Design review of the part built by this model. Coordinates are the model's own, in mm. Face numbers are marked on the shaded views. Round coordinates to 2 decimals unless told otherwise and drop trailing zeros. Order: outer loops, then holes, each group sorted by start corner. A loop starts at its lowest first (then second) coordinate and runs counter-clockwise, first axis right, second up.
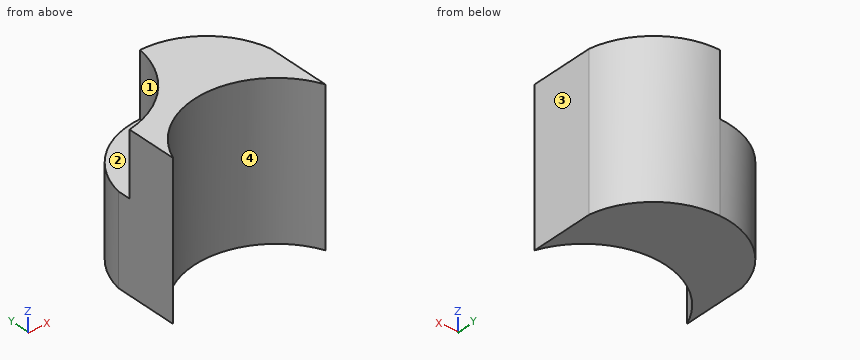
from build123d import *

# Parameters (mm, degrees)
SKETCH1_W           = 6
SKETCH1_H           = 6
BOSS_EXTRUDE1_DEPTH = 5
CUT_EXTRUDE4_DEPTH  = 12.5
CUT_EXTRUDE5_DEPTH  = 2.5


with BuildPart() as part:
    # Sketch1 → Boss-Extrude1 (new body)
    with BuildSketch(Plane(origin=(0, 0, 0), x_dir=(1, 0, 0), z_dir=(0, 1, 0))):
        Rectangle(SKETCH1_W, SKETCH1_H)
    extrude(amount=BOSS_EXTRUDE1_DEPTH)

    # Sketch5 → Cut-Extrude4 (cut)
    with BuildSketch(Plane.XY.offset(3)):
        with BuildLine():
            Line((-3, 5), (-3, 2.5))
            ThreePointArc((-3, 2.5), (-1.952562419, 4.293074903), (0, 5))
            Line((0, 5), (-3, 5))
        make_face()
        with BuildLine():
            ThreePointArc((0, 5), (1.952562419, 4.293074903), (3, 2.5))
            Line((3, 2.5), (3, 5))
            Line((3, 5), (0, 5))
        make_face()
        with BuildLine():
            ThreePointArc((-3, 0), (0, 2), (3, 0))
            Line((3, 0), (-3, 0))
        make_face()
    extrude(amount=-CUT_EXTRUDE4_DEPTH, mode=Mode.SUBTRACT)

    # Sketch6 → Cut-Extrude5 (cut)
    with BuildSketch(Plane.XY.offset(3)):
        with BuildLine():
            ThreePointArc((-3, 2), (-1.009831788, 3.009831788), (0, 5))
            ThreePointArc((0, 5), (-1.952562419, 4.293074903), (-3, 2.5))
            Line((-3, 2.5), (-3, 2))
        make_face()
    extrude(amount=-CUT_EXTRUDE5_DEPTH, mode=Mode.SUBTRACT)


solid = part.part
1) The part is to be moulded in two halves that separate along X. For the marked faces 1, 2, 3 and 4, say which applies: released by +X, released by -X, zero draft, split by the parting line, or undercut.
Results:
face 1: released by -X
face 2: zero draft
face 3: released by +X
face 4: undercut
2) To check wall thickness, follow line 1 along X through (y, z) = (1.1, 0.15) (3 decimals); line 2 along X through (y, z) = (1.55, 2.55); line 3 along Y through (x, z) = (2.5, -1.25). State the ranges of each line that lie inside material, in increasing order.
Results:
line 1: x = -3 to -2.245, 2.245 to 3
line 2: x = -3 to -1.65, 1.65 to 3
line 3: y = 0.83 to 3.7
3) Take a section at A-A on y = 0.4. Give the boundary of the cut face in (x, z).
Results:
outline: (-3, -3) - (-2.8, -3) - (-2.8, 3) - (-3, 3) - close; (2.8, -3) - (3, -3) - (3, 3) - (2.8, 3) - close
4) Take a section at B-B on z = -1. Give the boundary of the cut face in (x, y), plus the area to 3 significant figures.
Results:
outline: (-3, 0) arc R3.25 cw to (3, 0) - (3, 2.5) arc R3.05 ccw to (-3, 2.5) - close
area: 17.6 mm2
5) Take a section at D-D on y = 1.4. Give the boundary of the cut face in (x, z), plus the area to 3 significant figures.
Results:
outline: (-3, -3) - (-1.88, -3) - (-1.88, 3) - (-3, 3) - close; (1.88, -3) - (3, -3) - (3, 3) - (1.88, 3) - close
area: 13.4 mm2
6) Clearance check with a flat-ended pin moving along its axis: P1, Ø3, axis at x = 0.5, z = 1.5, coming from the -Y side. State where the tip first meets the part, or that it passes through.
Results:
P1: stops at y = 1.31
7) Take a section at C-C on x = -1. Give the boundary of the cut face in (y, z).
Results:
outline: (1.84, -3) - (4.83, -3) - (4.83, 0.5) - (3.02, 0.5) - (3.02, 3) - (1.84, 3) - close
